Can you work these out from the model? Positions are in its coordinate system, mm. Face numbers are marked on the shaded views. A direction names the side the tool comes from. Round coordinates to 2 decimals unless told otherwise and drop trailing zeros. Loops run counter-clockwise (first coordinate to the right, second up) from the corner with the lowest first, then second, coordinate; pieces in that order, holes last. Notation, with made-up numbers: (-34, 71.5) -> (-10, 71.5) arc R33 cw to (-10, 101.5) -> close; hole circle Ø9 at (21, 53). An arc over 180 degrees is marked (long way). Use a Markdown table: item, result.
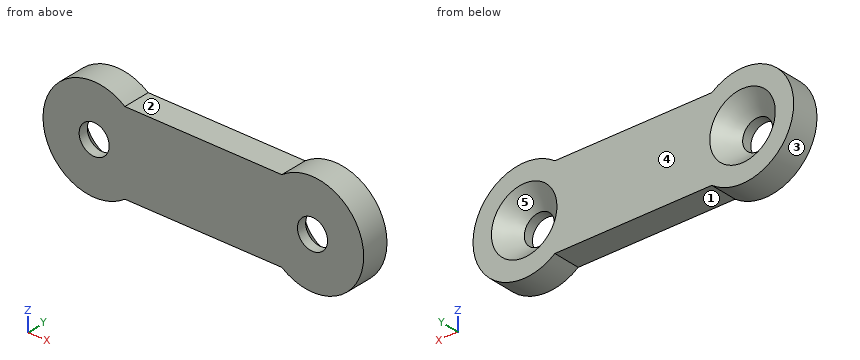
from build123d import *

# Parameters (mm, degrees)
SKETCH1_R           = 1.1
BOSS_EXTRUDE1_DEPTH = 2
BOSS_EXTRUDE3_START = -2
SKETCH3_R           = 3.75
SKETCH3_R_2         = 1.1
BOSS_EXTRUDE3_DEPTH = 2
CHAMFER1_SIZE       = 1.3


with BuildPart() as part:
    # Sketch1 → Boss-Extrude1 (new body)
    with BuildSketch(Plane(origin=(0, 0, 0), x_dir=(1, 0, 0), z_dir=(0, 1, 0))):
        with BuildLine():
            Line((-8, 3), (8, 3))
            ThreePointArc((8, 3), (11, 0), (8, -3))
            Line((8, -3), (-8, -3))
            ThreePointArc((-8, -3), (-11, 0), (-8, 3))
        make_face()
        with Locations(Location((-8, 0, 0), (0, 0, 270))):
            Circle(SKETCH1_R, mode=Mode.SUBTRACT)
        with Locations(Location((8, 0, 0), (0, 0, 270))):
            Circle(SKETCH1_R, mode=Mode.SUBTRACT)
    extrude(amount=BOSS_EXTRUDE1_DEPTH)

    # Sketch3 → Boss-Extrude3 (add)
    # profile 1 of 2: a face of its own
    with BuildSketch(Plane(origin=(0, 2, 0), x_dir=(1, 0, 0), z_dir=(0, 1, 0)).offset(BOSS_EXTRUDE3_START)):
        with Locations((-8, 0)):
            Circle(SKETCH3_R)
        with Locations(Location((-8, 0, 0), (0, 0, 270))):
            Circle(SKETCH3_R_2, mode=Mode.SUBTRACT)
    # profile 2 of 2: a face of its own
    with BuildSketch(Plane(origin=(0, 2, 0), x_dir=(1, 0, 0), z_dir=(0, 1, 0)).offset(BOSS_EXTRUDE3_START)):
        with Locations((8, 0)):
            Circle(SKETCH3_R)
        with Locations(Location((8, 0, 0), (0, 0, 270))):
            Circle(SKETCH3_R_2, mode=Mode.SUBTRACT)
    extrude(amount=BOSS_EXTRUDE3_DEPTH)

    # Chamfer1
    chamfer1_edges = [part.edges().sort_by_distance(p)[0] for p in [
        (-8, 2, -1.1),
        (8, 2, -1.1),
    ]]
    chamfer(chamfer1_edges, length=CHAMFER1_SIZE)


solid = part.part
1. Will these pins go through, and if not, where does the flat tip stop? pin 1 Ø0.6 at (x, y) = (0, 1.5) entering from -Z; pin 2 Ø2.5 at (x, z) = (8, 0) entering from +Y; pin 3 Ø0.6 at (x, y) = (-1.5, 1) entering from +Z.
Answer sheet:
| item | result |
|---|---|
| pin 1 | stops at z = -3 |
| pin 2 | stops at y = 0.85 |
| pin 3 | stops at z = 3 |
2. If we mould it in two halves opening along X, with no side actions, what happens to the marked faces 4 and 5? For each: +X half, -X half, draft (parallel to the pull), parting line (faces both ways), or undercut.
Answer sheet:
| item | result |
|---|---|
| face 4 | draft |
| face 5 | undercut |
3. I want a section at D-D (z = -3.25). Please give me the cut outline in (x, y), plus the area to 3 significant figures.
Answer sheet:
| item | result |
|---|---|
| outline | (-9.87, 0) -> (-6.13, 0) -> (-6.13, 2) -> (-9.87, 2) -> close; (6.13, 0) -> (9.87, 0) -> (9.87, 2) -> (6.13, 2) -> close |
| area | 15.0 mm² |
4. I need wall thicknesses on line 1 (X direction, y = 0.45, z = -0.5); line 2 (X direction, y = 1.5, z = -0.75); line 3 (Z direction, x = 1, y = 1.8). Which ranges of each line are inside material? Lowest first, please.
Answer sheet:
| item | result |
|---|---|
| line 1 | x = -11.72 to -8.98, -7.02 to 7.02, 8.98 to 11.72 |
| line 2 | x = -11.67 to -9.75, -6.25 to 6.25, 9.75 to 11.67 |
| line 3 | z = -3 to 3 |
5. I want a section at C-C (y = 1.75). Please give me the cut outline in (x, z), plus the area to 3 significant figures.
Answer sheet:
| item | result |
|---|---|
| outline | (-5.75, -3) -> (5.75, -3) arc R3.75 ccw (long way) to (5.75, 3) -> (-5.75, 3) arc R3.75 ccw (long way) to start; hole circle Ø4.3 at (-8, 0); hole circle Ø4.3 at (8, 0) |
| area | 116 mm² |
6. I want a section at A-A (x = 8). Please give me the cut outline in (y, z).
Answer sheet:
| item | result |
|---|---|
| outline | (0, -3.75) -> (2, -3.75) -> (2, -2.4) -> (0.7, -1.1) -> (0, -1.1) -> close; (0, 1.1) -> (0.7, 1.1) -> (2, 2.4) -> (2, 3.75) -> (0, 3.75) -> close |
7. Which directions (+Z, -Z, +X, -X, +Y, -Y) give clear straight access to the entire face, cutting with the end or side of a thin tool? Please do the marked faces 1, 2 and 3.
Answer sheet:
| item | result |
|---|---|
| face 1 | -Z, +Y, -Y |
| face 2 | +Z, +Y, -Y |
| face 3 | +Y, -Y |
8. I want a section at B-B (z = 0). Please give me the cut outline in (x, y).
Answer sheet:
| item | result |
|---|---|
| outline | (-11.75, 0) -> (-9.1, 0) -> (-9.1, 0.7) -> (-10.4, 2) -> (-11.75, 2) -> close; (-6.9, 0) -> (6.9, 0) -> (6.9, 0.7) -> (5.6, 2) -> (-5.6, 2) -> (-6.9, 0.7) -> close; (9.1, 0) -> (11.75, 0) -> (11.75, 2) -> (10.4, 2) -> (9.1, 0.7) -> close |
